Study the drawing (mm; zero at the part's minimum x, y, z) and answer. A direction names the side the tool comes from. Give positions to 0.01 mm unless a question says otherwise; leave off trailing zeros. Loops run counter-clockwise (first coordinate to the right, second up) from the corner with the lowest first, then second, coordinate; pieces in that order, holes last. Notation, with made-up numbers: (-8.5, 70) - (-4.5, 70) arc R20 cw to (-4.5, 101) - close; hole circle Ø1 at (53.5, 80). An arc over 180 degrees is marked (long way). Write item = value, one per line. Start each with the question number.
1) Consider probe 1 along X at (y, z) = (5.25, 2.25); probe 2 along X at (y, z) = (10.75, 5.5); probe 3 along X at (y, z) = (11.5, 25.25) (1 decimal). Determine where each line is inside the solid, lowest interval first.
2) Which of the six approach directions +Z, -Z, +X, -X, +Y, -Y give full straight-line access (tool end or side, diameter ignored) to the marked faces 4, 5, 6, 7 and 8?
3) The mould has two halves that part along X. Classify the marked faces 1, 2 and 3: +X half, -X half, draft (parallel to the pull), parting line (faces both ways), or undercut.
4) The part is cut by section A-A on y = 11.75. Write down the section's boundary in (x, z), plus the area to 3 significant figures.
5) The part is cut by section C-C on z = 13.25. Write down the section's boundary in (x, y).
6) The part is cut by section D-D on x = 3. Write down the section's boundary in (y, z).
7) The part is cut by section B-B on x = 9.75. Write down the section's boundary in (y, z).
8) Flat-ended cylindrical pins translate along their axes: P1, Ø4, axis at x = 10.5, y = 8, coming from the -Z side; P2, Ø0.6, axis at y = 4.5, z = 24, coming from the +X side; P3, Ø0.6, axis at y = 3.5, z = 24.5, coming from the -X side. Find the tip coordinate at first contact, or state that the pin passes through.
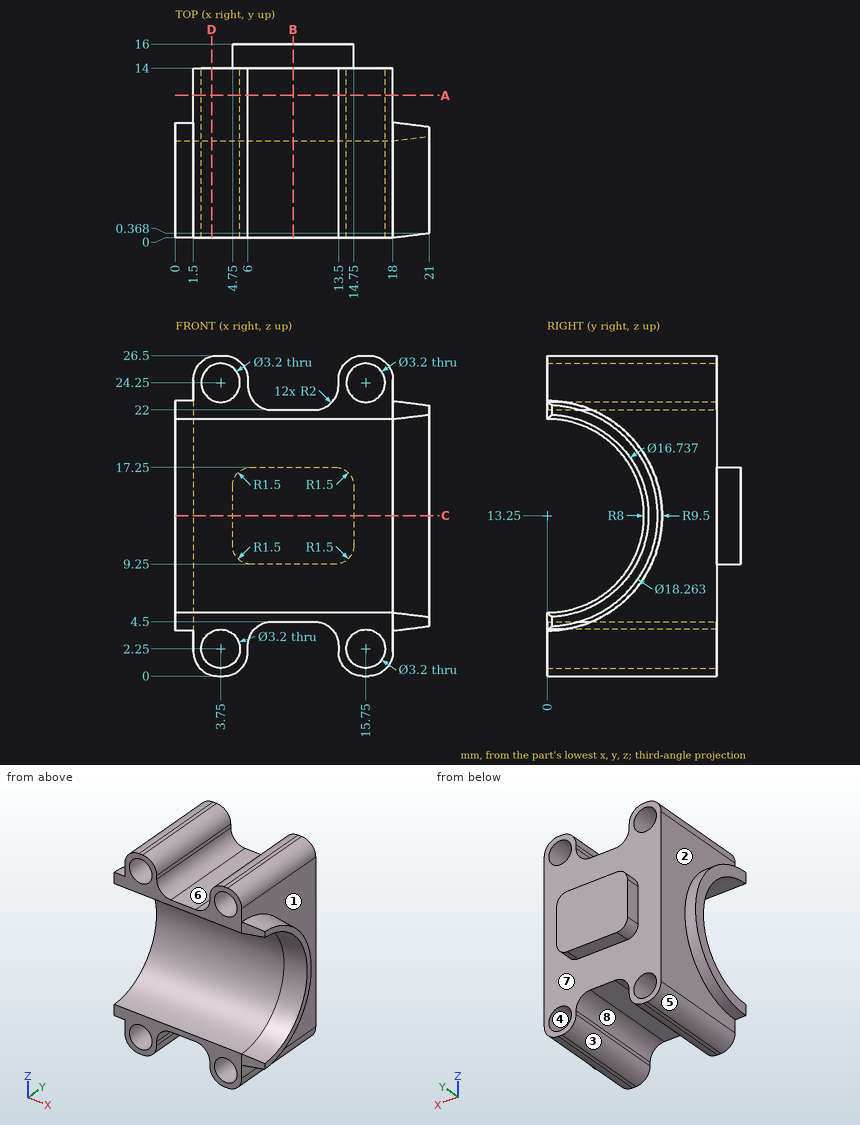
Answer below:
q1.probe_1 = 1.5 to 2.15, 5.35 to 6, 13.5 to 14.15, 17.35 to 18
q1.probe_2 = 1.5 to 18
q1.probe_3 = 1.6 to 2.5, 5 to 5.9, 13.6 to 14.5, 17 to 17.9
q2.face_4 = +Y, -Y
q2.face_5 = -Z, -X, +Y, -Y
q2.face_6 = +Z, +Y, -Y
q2.face_7 = +Y
q2.face_8 = -Z, +Y, -Y
q3.face_1 = +X half
q3.face_2 = -X half
q3.face_3 = undercut
q4.outline = (1.5, 2) arc R2 ccw to (3.5, 0) - (4, 0) arc R2 ccw to (6, 2) - (6, 2.5) arc R2 cw to (8, 4.5) - (11.5, 4.5) arc R2 cw to (13.5, 2.5) - (13.5, 2) arc R2 ccw to (15.5, 0) - (16, 0) arc R2 ccw to (18, 2) - (18, 24.5) arc R2 ccw to (16, 26.5) - (15.5, 26.5) arc R2 ccw to (13.5, 24.5) - (13.5, 24) arc R2 cw to (11.5, 22) - (8, 22) arc R2 cw to (6, 24) - (6, 24.5) arc R2 ccw to (4, 26.5) - (3.5, 26.5) arc R2 ccw to (1.5, 24.5) - close; hole circle Ø3.2 at (3.75, 2.25); hole circle Ø3.2 at (3.75, 24.25); hole circle Ø3.2 at (15.75, 2.25); hole circle Ø3.2 at (15.75, 24.25)
q4.area = 334 mm2
q5.outline = (0, 8) - (18, 8) - (21, 8.37) - (21, 9.13) - (18, 9.5) - (18, 14) - (14.75, 14) - (14.75, 16) - (4.75, 16) - (4.75, 14) - (1.5, 14) - (1.5, 9.5) - (0, 9.5) - close
q6.outline = (0, 0.06) - (14, 0.06) - (14, 0.84) - (0, 0.84) - close; (0, 3.66) - (14, 3.66) - (14, 22.84) - (0, 22.84) - (0, 21.25) arc R8 cw to (0, 5.25) - close; (0, 25.66) - (14, 25.66) - (14, 26.44) - (0, 26.44) - close
q7.outline = (0, 4.5) - (14, 4.5) - (14, 9.25) - (16, 9.25) - (16, 17.25) - (14, 17.25) - (14, 22) - (0, 22) - (0, 21.25) arc R8 cw to (0, 5.25) - close
q8.P1 = 4.23
q8.P2 = 18
q8.P3 = 1.5
